Source: CAD feature listing. Evaluate the final solid. Frame: model axes, mm. A direction names the side the tool comes from. Round coordinates to 2 decimals unless told otherwise and drop trailing zeros. Write each loop counter-clockwise with the first axis right and the second up, starting at its lowest first coordinate (ties: lowest second). Pieces come first, ordered by that corner, then holes. Notation, with made-up numbers: M 30.25,89.5 L 89.25,89.5 A37 cw 89.25,125.5 Z; hole C -4.75,87 d5. An arc over 180 degrees is marked long. Use a Markdown table: item, result.
```python
from build123d import *

# Parameters (mm, degrees)
SKETCH1_R           = 4
BOSS_EXTRUDE1_DEPTH = 40.72


with BuildPart() as part:
    # Sketch1 → Boss-Extrude1 (new body)
    with BuildSketch(Plane.XY):
        Polygon((40.7, -3.677490775), (40.7, -9.677490775), (-40.7, -9.677490775), (-40.7, -3.677490775), (-34.35, -3.677490775), (-34.35, 12.322509225), (-40.7, 12.322509225), (-40.7, 18.322509225), (40.7, 18.322509225), (40.7, 12.322509225), (34.35, 12.322509225), (34.35, -3.677490775), align=None)
        with Locations((20.35, 4.322509225)):
            Circle(SKETCH1_R, mode=Mode.SUBTRACT)
        with Locations(Location((-20.35, 4.322509225, 0), (0, 0, 180))):
            Circle(SKETCH1_R, mode=Mode.SUBTRACT)
    extrude(amount=-BOSS_EXTRUDE1_DEPTH)


solid = part.part
```
Q1. Section C-C on y = -1.25. Return loops of the section in (x, z).
Results are:
| item | result |
|---|---|
| outline | M -34.35,-40.72 L 34.35,-40.72 L 34.35,0 L -34.35,0 Z |
Q2. Section A-A on x = 20.35. Return loops of the section in (y, z).
Results are:
| item | result |
|---|---|
| outline | M -9.68,-40.72 L 0.32,-40.72 L 0.32,0 L -9.68,0 Z; M 8.32,-40.72 L 18.32,-40.72 L 18.32,0 L 8.32,0 Z |
Q3. Section B-B on z = -15.5. Return loops of the section in (x, y), plus the area to 3 significant figures.
Results are:
| item | result |
|---|---|
| outline | M -40.7,-9.68 L 40.7,-9.68 L 40.7,-3.68 L 34.35,-3.68 L 34.35,12.32 L 40.7,12.32 L 40.7,18.32 L -40.7,18.32 L -40.7,12.32 L -34.35,12.32 L -34.35,-3.68 L -40.7,-3.68 Z; hole C -20.35,4.32 d8; hole C 20.35,4.32 d8 |
| area | 1,980 mm^2 |
Q4. Reachability of faces 4 (the flat face through (-34.35, 4, -20)), 5 (the flat face through (38, 12.323, -20)), 6 (the flat face through (40.7, -7, -20)) from +Z, -Z, +X, -X, +Y, -Y: full face, straight path, thin tool, end or side. Return the list, or none.
Results are:
| item | result |
|---|---|
| face 4 | +Z, -Z, -X |
| face 5 | +Z, -Z, +X |
| face 6 | +Z, -Z, +X, +Y, -Y |
Q5. Mould query, pull axis Y, two halves, no side actions, for faces 1 (the flat face through (-40.7, -7, -20)), 2 (the flat face through (-1, 18.323, -20)), 3 (the flat face through (37, -3.677, -20)). Classes: +Y half, -Y half, draft (parallel to the pull), parting line (faces both ways), or undercut.
Results are:
| item | result |
|---|---|
| face 1 | draft |
| face 2 | +Y half |
| face 3 | undercut |
Q6. First-contact query: pin 1 Ø1.5 at (y, z) = (7, -24) entering from +X; pin 2 Ø13 at (x, y) = (20.35, 4.32) entering from -Z; pin 3 Ø5 at (y, z) = (4, -26.5) entering from -X. Flat tips, straight axial feed; report the tip coordinate or a pass-through.
Results are:
| item | result |
|---|---|
| pin 1 | x = 34.35 |
| pin 2 | z = -40.72 |
| pin 3 | x = -34.35 |
Q7. Line query: L1, parallel to X at y = 4, z = -34.5; L2, parallel to Y at x = -20, z = -16; L3, parallel to X at y = 2.75, z = -30. Output: solid intervals per line, ascending.
Results are:
| item | result |
|---|---|
| L1 | -34.35 to -24.34, -16.36 to 16.36, 24.34 to 34.35 |
| L2 | -9.68 to 0.34, 8.31 to 18.32 |
| L3 | -34.35 to -24.03, -16.67 to 16.67, 24.03 to 34.35 |
